Read the model definition and answer for the solid it produces. Units are mm, in the model's axes. A direction names the side the tool comes from. Round coordinates to 2 decimals unless told otherwise and drop trailing zeros. Loops run counter-clockwise (first coordinate to the right, second up) from the corner with the lowest first, then second, coordinate; pieces in that order, holes last. Notation, with made-up numbers: (67, 21.5) - (116, 21.5) arc R20 ccw to (116, 45.5) - close; hole circle Ø2 at (59, 1.5). An arc over 180 degrees is marked (long way). Use CSV: the item, a comma, the result in double quotes. Start each with the question number.
1. A tool of negligible diameter and unlimited length cuts with its end or side. For faces 4 (the flat face through (10, -2, 1.27)), 5 (the flat face through (0, -20.32, 1)), 6 (the flat face through (10, -3.175, 2)), from which of +Z, -Z, +X, -X, +Y, -Y can it reach the whole face along a straight path? Write none if from no direction.
2. Consider line 1 along Y through (x, z) = (-6, -1); line 2 along X through (y, z) = (-20.25, 1.5); line 3 along Z through (x, y) = (4.5, -6) (3 decimals). Determine where each line is inside the solid, lowest interval first.
3. Find section B-B (z = -3). Give the vertices of the cut face in (x, y) (1 decimal).
4. Find section C-C (x = 0). Give the vertices of the cut face in (y, z) (3 decimals), and give its area (3 significant figures).
5. Determine the mould class of faces 1 (the flat face through (0, -7.62, 1)), 2 (the flat face through (10, -2, -1.27)), 3 (the flat face through (0, -11, -3.81)) for opening direction Z: +Z half, -Z half, draft (parallel to the pull), parting line (faces both ways), or undercut.
6. Given pin 1 Ø2.5 at (y, z) = (-14, 1) entering from -X; pin 2 Ø0.6 at (x, z) = (-10.5, -2.5) entering from -Y (3 decimals); pin 3 Ø5 at (x, y) = (-4.5, -13) entering from +Z (3 decimals); pin 4 Ø2.5 at (x, z) = (1.5, -1.5) entering from +Y, each flat-ended and moving along its own axis, determine where each tip first touches the part or whether it passes through.
from build123d import *

# Parameters (mm, degrees)
F0_W     = 18.923
F0_H     = 6.985
F1_DEPTH = 22.86
F3_DEPTH = 0.635
F4_W     = 12.7
F4_H     = 12.7
F5_DEPTH = 5.08
F4_W_2   = 1.143
F4_H_2   = 3.175
F6_DEPTH = 6.985
F7_W     = 1.143
F7_H     = 2.54
F8_DEPTH = 12.7


# Not quite as in the source:
# - a feature names something its author has since deleted; it is built from what else it names


with BuildPart() as f1:
    # F0 (on Front) → F1 (new body)
    with BuildSketch(Plane.XZ):
        with Locations((0, -0.3175)):
            Rectangle(F0_W, F0_H)
    extrude(amount=F1_DEPTH)

    # F2 (on face) → F3 (join)
    with BuildSketch(Plane.XZ.offset(22.86)):
        Polygon((9.9764279214, 4.318), (-9.9695, 4.318), (-9.9695, -3.81), (-9.4615, -3.81), (-9.4615, 3.175), (9.4615, 3.175), (9.4615, -3.81), (9.9764279214, -3.81), align=None)
    extrude(amount=-F3_DEPTH)

    # F4 (on face) → F5 (cut)
    with BuildSketch(Plane.XY.offset(3.175)):
        with Locations((0, -13.97)):
            Rectangle(F4_W, F4_H)
    extrude(amount=-F5_DEPTH, mode=Mode.SUBTRACT)

    # F4 (on face) → F6 (join, through all)
    with BuildSketch(Plane.XY.offset(3.175)):
        with Locations((-10.033, -1.5875)):
            Rectangle(F4_W_2, F4_H_2)
        with Locations((10.033, -1.5875)):
            Rectangle(F4_W_2, F4_H_2)
    extrude(amount=-F6_DEPTH)

    # F7 (on face) → F8 (cut)
    with BuildSketch(Plane.XZ):
        with Locations((10.033, 0)):
            Rectangle(F7_W, F7_H)
        with Locations((-10.033, 0)):
            Rectangle(F7_W, F7_H)
    extrude(amount=F8_DEPTH, mode=Mode.SUBTRACT)


solid = f1.part
Filled sheet:
1,face 4,"+X, +Y"
1,face 5,"+Z"
1,face 6,"+Z, -Z, +X"
2,line 1,"y = -22.86 to -20.32, -7.62 to 0"
2,line 2,"x = -9.46 to -6.35, 6.35 to 9.46"
2,line 3,"z = -3.81 to 3.175"
3,outline,"(-10.6, -3.2) - (-9.5, -3.2) - (-9.5, -22.2) - (-10, -22.2) - (-10, -22.9) - (10, -22.9) - (10, -22.2) - (9.5, -22.2) - (9.5, -3.2) - (10.6, -3.2) - (10.6, 0) - (-10.6, 0) - close"
4,outline,"(-22.86, -3.81) - (0, -3.81) - (0, 3.175) - (-7.62, 3.175) - (-7.62, -1.905) - (-20.32, -1.905) - (-20.32, 3.175) - (-22.225, 3.175) - (-22.225, 4.318) - (-22.86, 4.318) - close"
4,area,"95.9 mm²"
5,face 1,"draft"
5,face 2,"undercut"
5,face 3,"-Z half"
6,pin 1,"stops at x = -9.46"
6,pin 2,"stops at y = -3.175"
6,pin 3,"stops at z = 3.175"
6,pin 4,"stops at y = 0"
